The model under review builds one solid part; all positions refer to its coordinate system, in mm. A direction names the side the tool comes from. Round coordinates to 2 decimals unless told otherwise and drop trailing zeros. Order: outer loops, then holes, each group sorted by start corner. A loop starts at its lowest first (then second) coordinate and runs counter-clockwise, first axis right, second up. Notation, with made-up numbers: M -23,26.25 L 25,26.25 A19 ccw 25,42.25 Z; hole C 34,-5.75 d6. An arc over 180 degrees is marked long. Answer as a JSON object with one key per item and string values. Group by question number.
1) Consider section D-D, the plane z = 47. Write out the cut boundary in (x, y).
2) Consider section C-C, the plane x = 40. Write out the cut boundary in (y, z).
3) Insertion check: pin 1 Ø8 at (x, y) = (37, 121) entering from +Z; pin 2 Ø1.5 at (x, y) = (75, 95.5) entering from +Z; pin 3 Ø10 at (x, z) = (133.5, 52.5) entering from -Y; pin 4 Ø16 at (x, z) = (110, 90) entering from -Y. Each pin has a flat end and moves straight along its axis. Give the tip position at first contact, or say it passes through.
4) For faces 1 (the flat face through (50, 80, 80)), 2 (the flat face through (32, 97, 100)), 3 (the flat face through (79, 101, 0)), list the 3-axis set-ups (+Z, -Z, +X, -X, +Y, -Y) from which the entire face can be reached by the end or side of a thin tool; tool diameter is ignored.
5) The part is to be moulded in two halves that separate along Y. For faces 4 (the flat face through (38, 0, 38)), 5 (the flat face through (81, 200, 59)), 6 (the flat face through (81, 180, 120)), 7 (the cylindrical face through (46, 138, 49)), say which applies: +Y half, -Y half, draft (parallel to the pull), parting line (faces both ways), or undercut.
6) Consider section A-A, the plane z = 84. Write out the cut boundary in (x, y), then the cut area to 3 significant figures.
7) Consider section B-B, the plane y = 130. Write out the cut boundary in (x, z), then the cut area to 3 significant figures.
8) To check wall thickness, follow line 1 (Y direction, x = 40, z = 35); line 2 (Z direction, x = 110, y = 186.5); line 3 (X direction, y = 130, z = 79). State the ranges of each line that lie inside material, in increasing order.
Autodesk Fusion 360 part; units mm, degrees
sketch "Sketch1" plane through (0, 0, 0) normal (0, 0, 1) x (1, 0, 0)
  line L0 (0, 0) -> (0, 200)
  line L1 (0, 200) -> (160, 200)
  line L2 (160, 200) -> (160, 60)
  line L3 (0, 0) -> (100, 0)
  line L4 (100, 0) -> (160, 60)
extrude "Extrude1" add sketch "Sketch1" along normal blind 60
sketch "Sketch2" plane through (0, 0, 60) normal (0, 0, 1) x (-1, 0, 0)
  line L0 (0, 0) -> (-100, 0)
  line L1 (-100, 0) -> (-160, -60)
  line L2 (-160, -60) -> (-160, -200)
  line L3 (-160, -200) -> (0, -200)
  line L4 (0, -200) -> (0, 0)
  line L5 (0, 0) -> (0, -160)
  line L6 (0, -160) -> (-80, -160)
  line L7 (-80, -160) -> (-80, -100)
  line L8 (0, 0) -> (-20, 0)
  line L9 (-20, 0) -> (-20, -60)
  line L10 (-20, -60) -> (-80, -100)
  line L11 (0, -160) -> (0, -200)
  line L12 (-160, -200) -> (-160, -180)
  line L13 (-160, -180) -> (-140, -160)
  line L14 (-140, -160) -> (-80, -160)
extrude "Extrude2" add sketch "Sketch2" along normal blind 40 contours L0 L4 L5 L6 L7 L8 L9 L10
extrude "Extrude3" add sketch "Sketch2" along normal blind 60 contours L2 L3 L4 L6 L11 L12 L13 L14
sketch "Sketch3" plane through (0, 160, 0) normal (0, -1, 0) x (1, 0, 0)
  line L0 (0, 100) -> (80, 100)
  line L1 (80, 100) -> (80, 60)
  line L2 (80, 60) -> (140, 60)
  line L3 (140, 60) -> (140, 120)
  line L4 (140, 120) -> (0, 120)
  line L5 (0, 120) -> (0, 100)
  circle A0 centre (110, 90) radius 10
  line L6 (110, 90) -> (110, 120)
  dimension "d17" = 20
hole "Hole1" at (110, 160, 90) direction (0, 1, 0) diameter 20 depth 40 tip angle 118
sketch "Sketch4" plane through (0, 0, 100) normal (0, 0, 1) x (-1, 0, 0)
  line L0 (0, 0) -> (-20, 0)
  line L1 (-20, 0) -> (-20, -60)
  line L2 (-20, -60) -> (-80, -100)
  line L3 (-80, -100) -> (-80, -160)
  line L4 (-80, -160) -> (0, -160)
  line L5 (0, -160) -> (0, 0)
hole "Hole2" at (40, 130, 100) direction (0, 0, -1) diameter 20 depth 1000 tip angle 118
Results list:
{
 "1": {"outline": "M 0,0 L 100,0 L 160,60 L 160,200 L 0,200 Z; hole C 40,130 d20"},
 "2": {"outline": "M 0,0 L 120,0 L 120,100 L 73.33,100 L 73.33,60 L 0,60 Z; M 140,0 L 200,0 L 200,120 L 160,120 L 160,100 L 140,100 Z"},
 "3": {"pin 1": "z = 100", "pin 2": "z = 60", "pin 3": "y = 28.5", "pin 4": "through"},
 "4": {"face 1": "+Z, +X, -Y", "face 2": "+Z, +X, -X, -Y", "face 3": "-Z, +X, -X, +Y, -Y"},
 "5": {"face 4": "-Y half", "face 5": "+Y half", "face 6": "draft", "face 7": "undercut"},
 "6": {"outline": "M 0,0 L 20,0 L 20,60 L 80,100 L 80,160 L 102,160 L 102,200 L 0,200 Z; M 118,160 L 140,160 L 160,180 L 160,200 L 118,200 Z; hole C 40,130 d20", "area": "13,200 mm^2"},
 "7": {"outline": "M 0,0 L 30,0 L 30,100 L 0,100 Z; M 50,0 L 160,0 L 160,60 L 80,60 L 80,100 L 50,100 Z", "area": "10,800 mm^2"},
 "8": {"line 1": "0 to 120, 140 to 200", "line 2": "0 to 80, 100 to 120", "line 3": "0 to 30, 50 to 80"}
}
